from build123d import *

# Parameters (mm, degrees)
F0_W     = 150
F0_H     = 86
F1_DEPTH = 140
F2_R     = 1.75
F3_DEPTH = 1


with BuildPart() as f1:
    # F0 (on Front) → F1 (new body)
    with BuildSketch(Plane.XZ):
        Rectangle(F0_W, F0_H)
    extrude(amount=F1_DEPTH)

    # F2 (on face) → F3 (cut)
    with BuildSketch(Plane(origin=(0, 0, 0), x_dir=(-1, 0, 0), z_dir=(0, 1, 0))):
        with Locations((-69, -37)):
            Circle(F2_R)
    extrude(amount=-F3_DEPTH, mode=Mode.SUBTRACT)


solid = f1.part
Geometry check sheet. Reference: the model listing, model coordinates, mm. A direction names the side the tool comes from. Give positions to 0.01 mm unless a question says otherwise; leave off trailing zeros.
1) Set-up check for faces 4 (the face through (-75, -69, -1)), 5 (the face through (69, -1, -37)): record each of +Z, -Z, +X, -X, +Y, -Y from which the full face is reachable in a straight line by a thin tool's end or side.
Values follow:
face 4: +Z, -Z, -X, +Y, -Y
face 5: +Y
2) Release check for a two-part mould opening along X. For faces 1 (the face through (75, -69, -1)), 2 (the face through (67.331, -0.493, -36.474)), 3 (the face through (-1, -140, 1)) record: released by +X, released by -X, zero draft, split by the parting line, or undercut.
Values follow:
face 1: released by +X
face 2: undercut
face 3: zero draft
3) Go/stop test with a flat-tipped pin: pin 1 Ø1 at (x, z) = (69, -38) entering from +Y. Record where the tip stops, or that it passes through.
Values follow:
pin 1: stops at y = -1
4) Thickness scan on line 1 (Z direction, x = 69, y = -0.7). Record the ranges inside material, lowest first.
Values follow:
line 1: z = -43 to -38.75, -35.25 to 43
